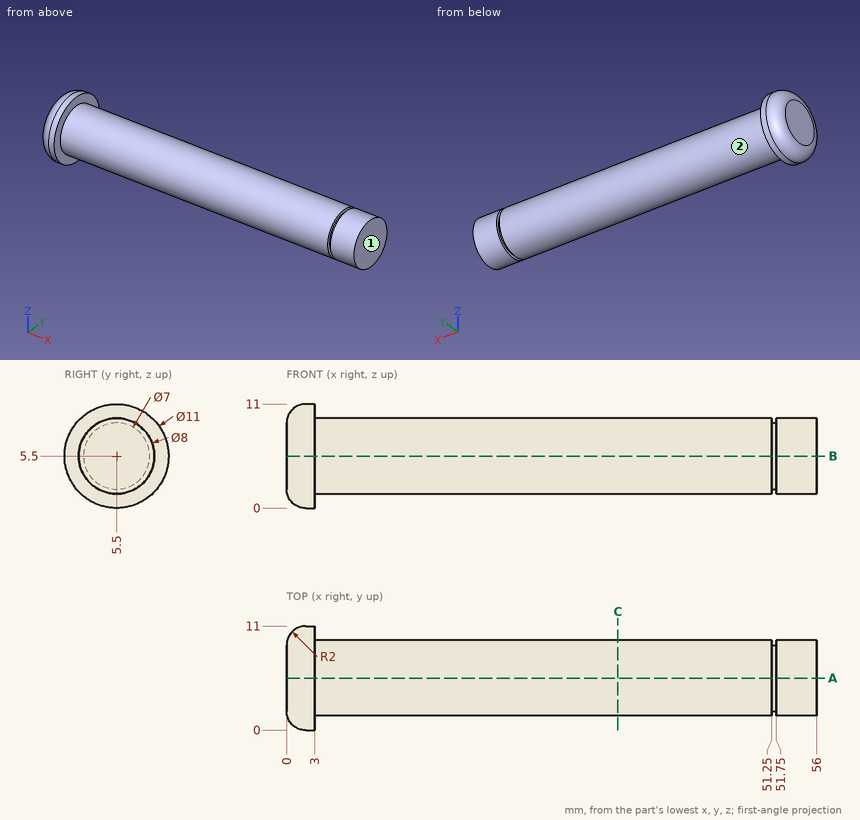
Study the drawing (mm; zero at the part's minimum x, y, z) and answer. A direction names the side the tool comes from. Coordinates: 2 decimals unless noted, no trailing zeros. Loops run counter-clockwise (first coordinate to the right, second up) from the corner with the lowest first, then second, coordinate; pieces in that order, holes last. Notation, with made-up numbers: (-27.75, 88.5) -> (12.25, 88.5) arc R27 cw to (12.25, 120.5) -> close; hole circle Ø1 at (38, -34.75). An arc over 180 degrees is marked (long way). Write each question's results on one line, items separated by ' | '. Start each with the question number.
1) For the marked faces 1 and 2, determine the directions among +Z, -Z, +X, -X, +Y, -Y from which every point of the face is accessible in a straight line to the end or side of a thin tool.
2) Find section A-A on y = 5.5. Determine the outline of the cut face in (x, z), then the cut area to 3 significant figures.
3) Find section C-C on x = 35. Determine the outline of the cut face in (y, z), then the cut area to 3 significant figures.
4) Flat-ended cylindrical pins translate along their axes: P1, Ø4, axis at x = 34, y = 1.5, coming from the -Z side; P2, Ø5, axis at x = 39.5, y = 4, coming from the -Z side; P3, Ø1.5, axis at y = 6.5, z = 6, coming from the -X side; P4, Ø1, axis at x = 19, y = 5.5, coming from the +Z side. Find the tip coordinate at first contact, or state that the pin passes through.
5) Consider line 1 along X through (y, z) = (6.5, 9.25); line 2 along Z through (x, y) = (23, 5.25); line 3 along X through (y, z) = (8, 1). Determine where each line is inside the solid, lowest interval first.
Response values:
1) face 1: +Z, -Z, +X, +Y, -Y | face 2: +X
2) outline: (0, 2) arc R2 ccw to (2, 0) -> (3, 0) -> (3, 1.5) -> (51.25, 1.5) -> (51.25, 2) -> (51.75, 2) -> (51.75, 1.5) -> (56, 1.5) -> (56, 9.5) -> (51.75, 9.5) -> (51.75, 9) -> (51.25, 9) -> (51.25, 9.5) -> (3, 9.5) -> (3, 11) -> (2, 11) arc R2 ccw to (0, 9) -> close | area: 455 mm^2
3) outline: circle Ø8 at (5.5, 5.5) | area: 50.3 mm^2
4) P1: stops at z = 2.04 | P2: stops at z = 1.5 | P3: stops at x = 0 | P4: stops at z = 9.5
5) line 1: x = 0.04 to 51.25, 51.75 to 56 | line 2: z = 1.51 to 9.49 | line 3: x = 0.87 to 3
